Could you check a few things on this model? Use its own coordinates, in mm. Face numbers are marked on the shaded views. A direction names the side the tool comes from. Round coordinates to 2 decimals unless told otherwise and drop trailing zeros. Loops run counter-clockwise (first coordinate to the right, second up) from the corner with the lowest first, then second, coordinate; pieces in that order, holes last. Notation, with made-up numbers: (-5, -3) -> (42, -3) arc R8 cw to (42, 5) -> close; hole circle Ø3 at (32.25, 22). An arc over 180 degrees is marked (long way). One line per item, written item: value.
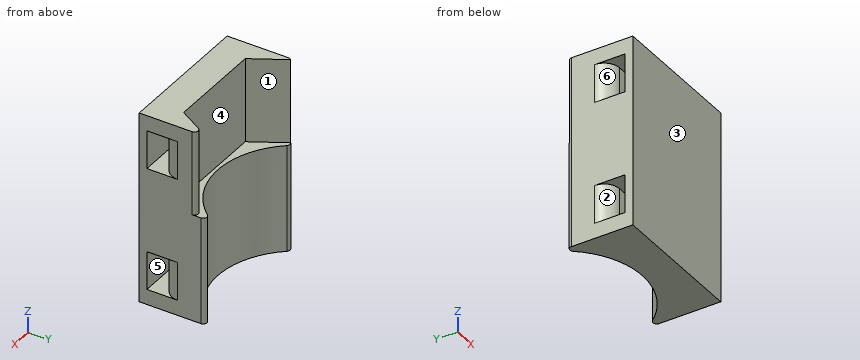
Autodesk Fusion 360 part; units mm, degrees
sketch "Sketch1" plane through (0, 0, 0) normal (0, 0, 1) x (1, 0, 0)
  circle A0 centre (0, 0) radius 10.5
  line L0 (-6.3076, 10.925) -> (-12.6151, 0)
  line L1 (-12.6151, 0) -> (-6.3076, -10.925)
  line L2 (-6.3076, -10.925) -> (6.3076, -10.925)
  line L3 (6.3076, -10.925) -> (12.6151, 0)
  line L4 (12.6151, 0) -> (6.3076, 10.925)
  line L5 (6.3076, 10.925) -> (-6.3076, 10.925)
  line L6 (-4.6188, 8) -> (-9.2376, 0)
  line L7 (-9.2376, 0) -> (-4.6188, -8)
  line L8 (-4.6188, -8) -> (4.6188, -8)
  line L9 (4.6188, -8) -> (9.2376, 0)
  line L10 (9.2376, 0) -> (4.6188, 8)
  line L11 (4.6188, 8) -> (-4.6188, 8)
  dimension "d2" = 21
  dimension "d3" = 10.925
  dimension "d15" = 8
extrude "Extrude2" add sketch "Sketch1" along normal blind 15 contours A0 | L6 L7 L8 L9 L10 L11 makes body 1
extrude "Extrude3" add sketch "Sketch1" along normal blind 12 from surface at 15 contours A0 | L0 L1 L2 L3 L4 L5 | L6 L7 L8 L9 L10 L11 bodies 1
extrude "Extrude4" add sketch "Sketch1" along normal blind 17 from surface at 27 contours L6 L7 L8 L9 L10 L11 bodies 1
sketch "Sketch2" plane through (0, 0, 0) normal (0, 1, 0) x (1, 0, 0)
  line L0 (-9, -1) -> (9, -1)
  line L1 (9, -1) -> (9, -26)
  line L2 (9, -26) -> (-9, -26)
  line L3 (-9, -26) -> (-9, -1)
extrude "Extrude5" add sketch "Sketch2" against normal blind 15 separate body makes body 2
combine "Combine1" operation cut target body 2 tool bodies 1 keep tools
sketch "Sketch3" plane through (9, 0, 0) normal (1, 0, 0) x (0, 1, 0)
  line L0 (-6.2615, 15) -> (-6.2615, 26)
  line L1 (-6.2615, 26) -> (-15, 26)
  line L2 (-15, 26) -> (-15, 1)
  line L3 (-15, 1) -> (-5.4083, 1)
  line L4 (-5.4083, 1) -> (-5.4083, 15)
  line L5 (-5.4083, 15) -> (-6.2615, 15)
  line L6 (-14, 24) -> (-12, 24)
  line L7 (-12, 24) -> (-12, 19)
  line L8 (-12, 19) -> (-14, 19)
  line L9 (-14, 19) -> (-14, 24)
  line L10 (-14, 3) -> (-12, 3)
  line L11 (-12, 3) -> (-12, 8)
  line L12 (-12, 8) -> (-14, 8)
  line L13 (-14, 8) -> (-14, 3)
  dimension "d24" = 2
  dimension "d25" = 5
  dimension "d26" = 2
  dimension "d27" = 5
  dimension "d28" = 2
  dimension "d29" = 2
extrude "Extrude6" cut sketch "Sketch3" against normal blind 28 contours L6 L7 L8 L9 | L10 L11 L12 L13 bodies 2
fillet "Fillet1" radius 2 4 edges at (9, -12, 21.5) (9, -12, 5.5) (-9, -12, 21.5) (-9, -12, 5.5) on bodies 2
fillet "Fillet2" radius 0.5 4 edges at (-9, -5.4083, 8) (-9, -6.2615, 20.5) (9, -6.2615, 20.5) (9, -5.4083, 8) on bodies 2
hidden bodies 1
equation "d3 = 21.85 mm / 2"
equation "d26 = d24"
equation "d27 = d25"
equation "d28 = d24"
equation "d29 = d24"
Item 1: If we section it at C-C on x = 1.75: List the corners of the cut face in (y, z) for me (3 decimals), plus the area to 3 significant figures.
Output:
outline: (-15, 1) -> (-10.353, 1) -> (-10.353, 15) -> (-10.925, 15) -> (-10.925, 26) -> (-15, 26) -> close; hole (-14, 3) -> (-12, 3) -> (-12, 8) -> (-14, 8) -> close; hole (-14, 19) -> (-12, 19) -> (-12, 24) -> (-14, 24) -> close
area: 89.9 mm²
Item 2: If we mould it in two halves opening along Y, with no side actions, what happens to the marked faces 1, 2 and 3? For each: released by +Y, released by -Y, zero draft, split by the parting line, or undercut.
Output:
face 1: released by +Y
face 2: undercut
face 3: released by -Y
Item 3: I need wall thicknesses on line 1 (Z direction, x = -2.75, y = -13); line 2 (Y direction, x = 0.25, z = 3.75); line 3 (Y direction, x = -3.75, z = 21.5) (3 decimals). Which ranges of each line are inside material? Lowest first, please. Write a range as from..to.
Output:
line 1: z = 1..3, 8..19, 24..26
line 2: y = -15..-14, -12..-10.5
line 3: y = -15..-14, -12..-10.925
Item 4: Will these pins go through, and if not, where does the flat tip stop? pin 1 Ø2.5 at (x, z) = (-4, 4.5) entering from +Y; pin 2 Ø9 at (x, z) = (3, 22.5) entering from +Y; pin 3 Ø2.5 at (x, z) = (-2, 22.5) entering from +Y (3 decimals).
Output:
pin 1: stops at y = -9.09
pin 2: stops at y = -8.86
pin 3: stops at y = -10.925
Item 5: If we section it at D-D on z = 12: List the corners of the cut face in (x, y) for me, plus the area to 3 significant figures.
Output:
outline: (-9, -15) -> (9, -15) -> (9, -6.98) arc R0.5 ccw to (8.11, -6.66) arc R10.5 cw to (-8.11, -6.66) arc R0.5 ccw to (-9, -6.98) -> close
area: 107 mm²
Item 6: If we section it at A-A on z = 20.5: List the corners of the cut face in (x, y) for me (3 decimals), plus the area to 3 significant figures.
Output:
outline: (-9, -15) -> (9, -15) -> (9, -14) -> (-9, -14) -> close; (-9, -10) arc R2 ccw to (-7, -12) -> (7, -12) arc R2 ccw to (9, -10) -> (9, -8.128) arc R0.5 ccw to (8.067, -7.878) -> (6.308, -10.925) -> (-6.308, -10.925) -> (-8.81, -6.59) arc R0.5 ccw to (-9, -6.982) -> close
area: 47.5 mm²
Item 7: If we section it at B-B on y = -13.25: List the corners of the cut face in (x, z) for me, plus the area to 3 significant figures.
Output:
outline: (-9, 1) -> (9, 1) -> (9, 3) -> (-9, 3) -> close; (-9, 8) -> (9, 8) -> (9, 19) -> (-9, 19) -> close; (-9, 24) -> (9, 24) -> (9, 26) -> (-9, 26) -> close
area: 270 mm²
Item 8: For the marked faces 4, 5 and 6, which set-ups out of +Z, -Z, +X, -X, +Y, -Y let a thin tool reach every point of the face, with its end or its side?
Output:
face 4: +Z, +Y
face 5: +X, -X
face 6: -X
